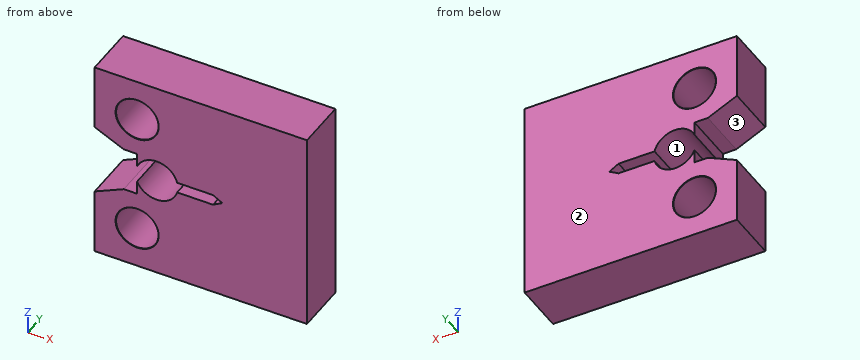
```python
from build123d import *

# Parameters (mm, degrees)
F0_R     = 6.25
F1_DEPTH = 7.5
F3_SIZE  = 0.1


with BuildPart() as f1:
    # F0 (on Front) → F1 (new body, symmetric)
    with BuildSketch(Plane.XZ):
        with BuildLine():
            ThreePointArc((-0.04, 0.0692820323), (-0.0107179677, 0.04), (0, 0))
            Line((0, 0), (14.3022312224, 0))
            Line((14.3022312224, 0), (25, 0))
            Line((25, 0), (25, 30))
            Line((25, 30), (-37.5, 30))
            Line((-37.5, 30), (-37.5, 10.5))
            Line((-37.5, 10.5), (-28.921972318, 6.5))
            Line((-28.921972318, 6.5), (-25, 6.5))
            Line((-25, 6.5), (-25, 2.5))
            ThreePointArc((-25, 2.5), (-18.7823742649, 6.2308090689), (-13.2234851669, 1.575))
            Line((-13.2234851669, 1.575), (-2.6479800219, 1.575))
            Line((-2.6479800219, 1.575), (-0.04, 0.0692820323))
        make_face()
        with Locations((-25, 17.75)):
            Circle(F0_R, mode=Mode.SUBTRACT)
    extrude(amount=F1_DEPTH, both=True)

    # F2: F1 across face


with BuildPart() as f1_1:
    add(f1.part)
    add(f1.part.mirror(Plane(origin=(12.5, 0, 0), x_dir=(1, 0, 0), z_dir=(0, 0, -1))))

    # F3
    f3_edges = [f1_1.edges().sort_by_distance(p)[0] for p in [
        (-31.25, -7.5, 17.75),
        (-31.25, -7.5, -17.75),
        (-31.25, 7.5, 17.75),
        (-31.25, 7.5, -17.75),
    ]]
    chamfer(f3_edges, length=F3_SIZE)


solid = f1_1.part
```
Source: CAD feature listing. Evaluate the final solid. Frame: model axes, mm. Face numbers are marked on the shaded views. A direction names the side the tool comes from. Give positions to 0.01 mm unless a question says otherwise; leave off trailing zeros. Order: outer loops, then holes, each group sorted by start corner. A loop starts at its lowest first (then second) coordinate and runs counter-clockwise, first axis right, second up.
(1) Material intervals for line 1 along Z through (x, y) = (-19.5, -6.25); line 2 along X through (y, z) = (2.5, -17.75); line 3 along Z through (x, y) = (-8, 1.5) (3 decimals), sorted ascending.
(2) Section query B-B (y = 6). Return the cut outline in (x, z) (3 decimals).
(3) Contact query for flat-ended pins moving along their axis: P1, Ø1, axis at y = -5.5, z = -2.5, coming from the -X side; P2, Ø10, axis at x = -31, z = -2, coming from the +Y side. Output: stop coordinate, or through.
(4) Section query C-C (x = -16). Return the cut outline in (y, z), plus the area to 3 significant figures.
(5) Section query D-D (z = 5). Return the cut outline in (x, y).
(6) Section query A-A (z = 17.75). Return the cut outline in (x, y).
(7) Access query for the marked faces 1, 2 and 3. Directions: +Z, -Z, +X, -X, +Y, -Y. A direction counts if a zero-diameter tool reaches every point of the face in a straight line with its end or side. Return the directions, or none.
Outcome:
1. line 1: z = -30 to -20.72, -14.78 to -6.25, 6.25 to 14.78, 20.72 to 30
1. line 2: x = -37.5 to -31.25, -18.75 to 25
1. line 3: z = -30 to -1.575, 1.575 to 30
2. outline: (-37.5, -30) - (25, -30) - (25, 30) - (-37.5, 30) - (-37.5, 10.5) - (-28.922, 6.5) - (-25, 6.5) - (-25, 2.5) arc R6.25 cw to (-13.223, 1.575) - (-2.648, 1.575) - (-0.04, 0.069) arc R0.08 cw to (-0.04, -0.069) - (-2.648, -1.575) - (-13.223, -1.575) arc R6.25 cw to (-25, -2.5) - (-25, -6.5) - (-28.922, -6.5) - (-37.5, -10.5) - close; hole circle Ø12.5 at (-25, -17.75); hole circle Ø12.5 at (-25, 17.75)
3. P1: stops at x = -25
3. P2: stops at y = 7.5
4. outline: (-7.5, -30) - (7.5, -30) - (7.5, -5.33) - (-7.5, -5.33) - close; (-7.5, 5.33) - (7.5, 5.33) - (7.5, 30) - (-7.5, 30) - close
4. area: 740 mm2
5. outline: (-25, -7.5) - (-23.02, -7.5) - (-23.02, 7.5) - (-25, 7.5) - close; (-15.52, -7.5) - (25, -7.5) - (25, 7.5) - (-15.52, 7.5) - close
6. outline: (-37.5, -7.5) - (-31.35, -7.5) - (-31.25, -7.4) - (-31.25, 7.4) - (-31.35, 7.5) - (-37.5, 7.5) - close; (-18.75, -7.4) - (-18.65, -7.5) - (25, -7.5) - (25, 7.5) - (-18.65, 7.5) - (-18.75, 7.4) - close
7. face 1: +Y, -Y
7. face 2: +Z, -Z, +X, -X, +Y
7. face 3: -X, +Y, -Y
